Design review of the part built by this model. Coordinates are the model's own, in mm. Face numbers are marked on the shaded views. Round coordinates to 2 decimals unless told otherwise and drop trailing zeros. Order: outer loops, then holes, each group sorted by start corner. A loop starts at its lowest first (then second) coordinate and runs counter-clockwise, first axis right, second up. Notation, with made-up numbers: (23.25, 68.5) - (71.25, 68.5) arc R22 ccw to (71.25, 102.5) - close; hole circle Ø4 at (44.25, 71). An arc over 180 degrees is marked (long way). Write item = value, one per line.
from build123d import *

# Parameters (mm, degrees)
SKETCH011_R             = 1.224307
PAD008_DEPTH            = 1
PAD009_DEPTH            = 2
SKETCH013_R             = 0.669574
PAD010_DEPTH            = 0.3
SKETCH014_W             = 3.347854
SKETCH014_H             = 4.253745
SKETCH014_W_2           = 3.426628
SKETCH014_H_2           = 4.174973
PAD011_DEPTH            = 2.5
PAD012_DEPTH            = 0.5
SKETCH016_R             = 2.3619034919
SKETCH016_R_2           = 2.482744
SKETCH016_W             = 2.528995
SKETCH016_H             = 10.003113
SKETCH016_W_2           = 9.696317
SKETCH016_H_2           = 9.027602
PAD013_DEPTH            = 1
PAD013_FACE69_W         = 9.027602
PAD013_FACE69_H         = 9.696317
PAD014_DEPTH            = 2
SKETCH017_R             = 1.308105
PAD015_DEPTH            = 2
SKETCH018_R             = 0.7
POCKET002_DEPTH         = 2
FILLET_R                = 0.6
FILLET001_R             = 1
BODY002_PLACEMENT_ANGLE = 180


with BuildPart() as part:
    # Sketch011 → Pad008 (new body)
    with BuildSketch(Plane.XY):
        Polygon((-64.871361, 16.524712), (-64.953331, -12.782201), (-64.465881, -13.950911), (-63.050274, -14.556654), (-9.769273, -14.098216), (-8.39049, -13.460031), (-7.653603, -12.197431), (-7.802202, -2.917618), (-30.061977, 19.617523), (-38.753654, 19.617523), (-38.912724, 18.463722), (-39.367214, 17.569231), (-63.35894, 17.690104), (-64.199226, 17.178921), align=None)
        with Locations((-60.089397, -9.239854)):
            Circle(SKETCH011_R, mode=Mode.SUBTRACT)
        with Locations((-31.335621, -9.166426)):
            Circle(SKETCH011_R, mode=Mode.SUBTRACT)
        with Locations((-36.552418, 17.295319)):
            Circle(SKETCH011_R, mode=Mode.SUBTRACT)
    extrude(amount=PAD008_DEPTH)

    # Sketch012 (on Face19 of Pad008) → Pad009 (join)
    with BuildSketch(Plane.XY.offset(1)):
        Polygon((-27.986155, 20.438019), (-35.378761, 14.19105), (-28.756979, 7.002593), (-21.645378, 13.573798), align=None)
        Polygon((-17.547031, 10.170015), (-30.422066, -1.999235), (-30.712292, -2.998892), (-21.228363, -13.603945), (-20.06669, -13.603945), (-6.912658, -1.370249), align=None)
    extrude(amount=PAD009_DEPTH)

    # Sketch013 (on Face5 of Pad009) → Pad010 (join)
    with BuildSketch(Plane.XY.offset(1)):
        with Locations((-55.712467, 16.086485)):
            Circle(SKETCH013_R)
        with Locations((-51.813202, 15.968324)):
            Circle(SKETCH013_R)
        with Locations((-47.913937, 15.928938)):
            Circle(SKETCH013_R)
        with Locations((-44.054054, 15.928938)):
            Circle(SKETCH013_R)
        with Locations((-40.115402, 15.889551)):
            Circle(SKETCH013_R)
        with Locations((-55.731503, 12.103284)):
            Circle(SKETCH013_R)
        with Locations((-51.832238, 11.985123)):
            Circle(SKETCH013_R)
        with Locations((-47.932973, 11.945737)):
            Circle(SKETCH013_R)
        with Locations((-44.07309, 11.945737)):
            Circle(SKETCH013_R)
        with Locations((-40.134438, 11.90635)):
            Circle(SKETCH013_R)
        with Locations((-55.668774, 8.025242)):
            Circle(SKETCH013_R)
        with Locations((-51.769509, 7.907081)):
            Circle(SKETCH013_R)
        with Locations((-47.870244, 7.867695)):
            Circle(SKETCH013_R)
        with Locations((-44.010361, 7.867695)):
            Circle(SKETCH013_R)
        with Locations((-40.071709, 7.828308)):
            Circle(SKETCH013_R)
        with Locations((-55.539787, -0.197736)):
            Circle(SKETCH013_R)
        with Locations((-51.640522, -0.315897)):
            Circle(SKETCH013_R)
        with Locations((-47.741257, -0.355283)):
            Circle(SKETCH013_R)
        with Locations((-43.881374, -0.355283)):
            Circle(SKETCH013_R)
        with Locations((-39.942722, -0.39467)):
            Circle(SKETCH013_R)
    extrude(amount=PAD010_DEPTH)

    # Sketch014 (on Face5 of Pad010) → Pad011 (join)
    with BuildSketch(Plane.XY.offset(1)):
        with Locations((-53.546768, -11.2506735)):
            Rectangle(SKETCH014_W, SKETCH014_H)
        with Locations((-40.746143, -11.0143545)):
            Rectangle(SKETCH014_W_2, SKETCH014_H_2)
    extrude(amount=PAD011_DEPTH)

    # Sketch015 (on Face66 of Pad011) → Pad012 (join)
    with BuildSketch(Plane.XY.offset(3.5)):
        with BuildLine():
            ThreePointArc((-52.61041275, -10.555223), (-53.57645, -9.58918575), (-54.54248725, -10.555223))
            Line((-54.54248725, -10.555223), (-54.54248725, -11.670621))
            ThreePointArc((-54.54248725, -11.670621), (-53.57645, -12.63665825), (-52.61041275, -11.670621))
            Line((-52.61041275, -10.555223), (-52.61041275, -11.670621))
        make_face()
        with BuildLine():
            ThreePointArc((-39.731315, -10.371226), (-40.628685, -9.473856), (-41.526055, -10.371226))
            Line((-41.526055, -10.371226), (-41.526055, -11.476269))
            ThreePointArc((-41.526055, -11.476269), (-40.628685, -12.373639), (-39.731315, -11.476269))
            Line((-39.731315, -10.371226), (-39.731315, -11.476269))
        make_face()
    extrude(amount=PAD012_DEPTH)

    # Sketch016 (on Face4 of Pad012) → Pad013 (join)
    with BuildSketch(Plane(origin=(0, 0, 0), x_dir=(1, 0, 0), z_dir=(0, 0, -1))):
        with Locations((-62.514374, 4.399912)):
            Circle(SKETCH016_R)
        with Locations((-62.376751, -12.940672)):
            Circle(SKETCH016_R_2)
        with Locations((-62.3010235, -4.3245135)):
            Rectangle(SKETCH016_W, SKETCH016_H)
        with Locations((-13.0114165, 8.686791)):
            Rectangle(SKETCH016_W_2, SKETCH016_H_2)
    extrude(amount=PAD013_DEPTH)

    # Pad013 Face69 → Pad014 (add)
    with BuildSketch(Plane(origin=(-13.0114165, -8.686791, -1), x_dir=(0, -1, 0), z_dir=(0, 0, -1))):
        Rectangle(PAD013_FACE69_W, PAD013_FACE69_H)
    extrude(amount=PAD014_DEPTH)

    # Sketch017 (on Face73 of Pad014) → Pad015 (join)
    with BuildSketch(Plane(origin=(0, 0, -1), x_dir=(1, 0, 0), z_dir=(0, 0, -1))):
        with Locations((-62.513016, 4.396934)):
            Circle(SKETCH017_R)
        with Locations((-62.376751, -12.940672)):
            Circle(SKETCH017_R)
    extrude(amount=PAD015_DEPTH)

    # Sketch018 (on Face114 of Pad015) → Pocket002 (cut)
    with BuildSketch(Plane(origin=(0, 0, -3), x_dir=(1, 0, 0), z_dir=(0, 0, -1))):
        with Locations((-62.513016, 4.396934)):
            Circle(SKETCH018_R)
        with Locations((-62.376751, -12.940672)):
            Circle(SKETCH018_R)
    extrude(amount=-POCKET002_DEPTH, mode=Mode.SUBTRACT)

    # Fillet
    fillet_edges = [part.edges().sort_by_distance(p)[0] for p in [
        (-13.489674, -7.487097, 3),
        (-23.984549, 4.08539, 3),
        (-25.970328, -8.301419, 3),
        (-30.567179, -2.499064, 3),
        (-20.647527, -13.603945, 3),
    ]]
    fillet(fillet_edges, radius=FILLET_R)

    # Fillet001
    fillet001_edges = [part.edges().sort_by_distance(p)[0] for p in [
        (-31.682458, 17.314535, 3),
        (-25.201179, 10.288196, 3),
    ]]
    fillet(fillet001_edges, radius=FILLET001_R)


with BuildPart() as part_1:
    # Body002 placement: moved
    add(part.part.moved(Location((1, -3.3, -5.7))).rotate(Axis((1, -3.3, -5.7), (1, 0, 0)), BODY002_PLACEMENT_ANGLE))


solid = part_1.part
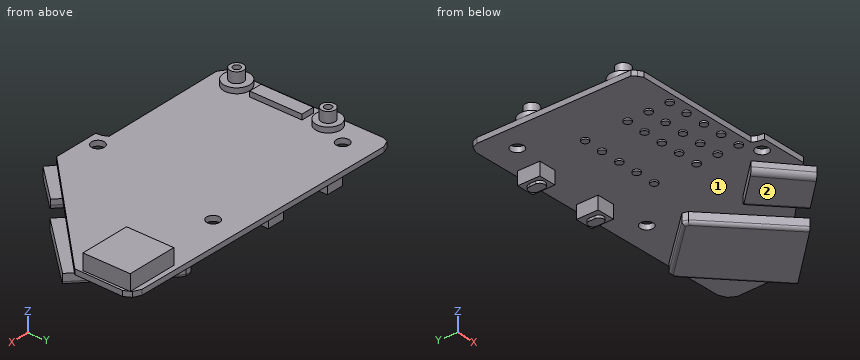
1) The part is to be moulded in two halves that separate along X. For the marked faces 1 and 2, say which applies: released by +X, released by -X, zero draft, split by the parting line, or undercut.
Findings:
face_1 = undercut
face_2 = zero draft
2) Clearance check with flat-ended pins moving along their axes: pin 1 Ø1 at (x, z) = (-40.5, -6.5) entering from +Y; pin 2 Ø2 at (x, y) = (-48.5, -7) entering from -Z; pin 3 Ø1.5 at (x, z) = (-11, -4.5) entering from +Y; pin 4 Ø0.8 at (x, z) = (-61.5, -5.5) entering from +Y. State where each tip first meets the part, or that it passes through.
Findings:
pin_1 = 11.08
pin_2 = -6.7
pin_3 = 9.9
pin_4 = 11.25
3) To check wall thickness, follow L1, parallel to X at y = 6, z = -5.75; L2, parallel to X at y = 8, z = -6.75; L3, parallel to Z at x = -46, y = 3. State the ranges of each line that lie inside material, in increasing order. Write a range as from..to.
Findings:
L1 = -63.94..-60.31, -57.87..-31.55, -29.12..-6.7
L2 = -54.22..-50.87, -41.46..-38.03, -22.29..-16.59
L3 = -6.7..-5.7
4) We need section A-A on x = -43. Write out the cut boundary in (y, z).
Findings:
outline = (-20.89, -6.7) - (-19.9, -6.7) - (-19.9, -7) - (-18.56, -7) - (-18.56, -6.7) - (-15.91, -6.7) - (-15.91, -7) - (-14.58, -7) - (-14.58, -6.7) - (-11.84, -6.7) - (-11.84, -7) - (-10.5, -7) - (-10.5, -6.7) - (-3.6, -6.7) - (-3.6, -7) - (-2.29, -7) - (-2.29, -6.7) - (11.09, -6.7) - (11.09, -5.7) - (-20.89, -5.7) - close
